from build123d import *

# Parameters (mm, degrees)
CHAMFER_4_SIZE = 1


with BuildPart() as part:
    # Эскиз1 → Повернуть1 (revolve)
    with BuildSketch(Plane.XY, mode=Mode.PRIVATE) as revolve_1_sk:
        Polygon((0, 5), (0, 28.5), (20, 28.5), (20, 23.2), (25, 23.2), (25, 22), (50, 22), (50, 23.2), (55, 23.2), (55, 5), align=None)
    revolve(revolve_1_sk.sketch.rotate(Axis((0, 0, 0), (1, 0, 0)), 90), axis=Axis((0, 0, 0), (1, 0, 0)))

    # Фаска4
    chamfer_4_edges = [part.edges().sort_by_distance(p)[0] for p in [
        (55, 0, -23.2),
        (55, 0, -5),
        (0, 0, -5),
        (0, 0, -28.5),
        (20, 0, -28.5),
    ]]
    chamfer(chamfer_4_edges, length=CHAMFER_4_SIZE)


solid = part.part
The listing builds one solid part. Answer for the finished solid, in the listing's coordinates (mm). A direction names the side the tool comes from. Round coordinates to 2 decimals unless told otherwise and drop trailing zeros. Order: outer loops, then holes, each group sorted by start corner. A loop starts at its lowest first (then second) coordinate and runs counter-clockwise, first axis right, second up. Notation, with made-up numbers: M -36,54 L -16,54 A29 ccw -16,85 Z; hole C 76.25,21.25 d11. An arc over 180 degrees is marked long. Answer in a Markdown table with one row per item. Add a question column.
1) Which of the six approach directions +Z, -Z, +X, -X, +Y, -Y give full straight-line access (tool end or side, diameter ignored) to faces 1 (the face through (25, 21, 8)), 2 (the face through (55, 5, 5)), 3 (the face through (52.028, -1.02, -23.178))?
2) Consider line 1 along Y through (x, z) = (24, 0); line 2 along Y through (x, z) = (16, 0); line 3 along X through (y, z) = (-1, 25). Determine where each line is inside the solid, lowest interval first. Write a range as from..to.
3) Flat-ended cylindrical pins translate along their axes: pin 1 Ø2 at (x, z) = (44.5, -6.5) entering from -Y; pin 2 Ø2 at (x, z) = (45, 10.5) entering from -Y; pin 3 Ø5 at (x, y) = (24.5, -9.5) entering from +Z. Find the tip coordinate at first contact, or state that the pin passes through.
4) Determine the mould class of faces 4 (the face through (20, 20.2, -12.4)), 5 (the face through (22.535, -1.02, -23.178)), 6 (the face through (50, 21, -8)) for opening direction X: pulls with the +X half, pulls with the -X half, needs draft (parallel to the pull), parting line crosses it, or undercut.
5) The part is cut by section D-D on x = 35. Determine the outline of the cut face in (y, z).
6) The part is cut by section C-C on x = 51.5. Determine the outline of the cut face in (y, z), plus the area to 3 significant figures.
Findings below:
| question | item | result |
|---|---|---|
| 1 | face 1 | none |
| 1 | face 2 | +Z, -Z, +X, +Y, -Y |
| 1 | face 3 | +X |
| 2 | line 1 | y = -23.2..-5, 5..23.2 |
| 2 | line 2 | y = -28.5..-5, 5..28.5 |
| 2 | line 3 | x = 0..20 |
| 3 | pin 1 | stops at y = -21.3 |
| 3 | pin 2 | stops at y = -19.84 |
| 3 | pin 3 | stops at z = 22.12 |
| 4 | face 4 | pulls with the +X half |
| 4 | face 5 | needs draft |
| 4 | face 6 | undercut |
| 5 | outline | C 0,0 d44; hole C 0,0 d10 |
| 6 | outline | C 0,0 d46.4; hole C 0,0 d10 |
| 6 | area | 1,610 mm² |
